Source: CAD feature listing. Evaluate the final solid. Frame: model axes, mm. Face numbers are marked on the shaded views. A direction names the side the tool comes from. Give positions to 0.01 mm unless a question says otherwise; leave off trailing zeros. Order: outer loops, then holes, each group sorted by start corner. A loop starts at its lowest first (then second) coordinate and runs counter-clockwise, first axis right, second up.
from build123d import *

# Parameters (mm, degrees)
SKETCH1_R                           = 66.675
FLANGE_DEPTH                        = 12.7
BOLT_HOLES_D                        = 6.35
BOLT_HOLES_DEPTH                    = 12.7
PIN_HOLES_D                         = 6.35
PIN_HOLES_DEPTH                     = 6.35
PIN_HOLES_TIP                       = 1.907732465
SKETCH2_R                           = 23.8125
SKETCH2_R_2                         = 12.7
FLOW_EXTRUDE_DEPTH                  = 12.7
SKETCH6_R                           = 13.081
SKETCH6_R_2                         = 4.7625
NITROUS_CONNECTION_FLANGE_DEPTH     = 12.7
SKETCH12_R                          = 23.8125
INITIAL_ENTRY_IMPINGING_PLATE_DEPTH = 5.715
SKETCH14_R                          = 23.749
SKETCH15_R                          = 23.8125
SKETCH16_R                          = 12.7
FINAL_FLOW_CUT_DEPTH                = 6.35
TAP_HOLES_FOR_IMPINGING_PLATE_D     = 3.7973
TAP_HOLES_FOR_IMPINGING_PLATE_DEPTH = 12.7
TAP_HOLES_FOR_IMPINGING_PLATE_TIP   = 1.140824014
FLOW_EXTRUDE_FILLET_R               = 3.175
FINAL_FILLET_FOR_HANDLING_R         = 0.635


with BuildPart() as part:
    # Sketch1 → Flange (new body)
    with BuildSketch(Plane(origin=(0, 0, 0), x_dir=(1, 0, 0), z_dir=(0, 1, 0))):
        Circle(SKETCH1_R)
    extrude(amount=FLANGE_DEPTH)

    # Bolt Holes
    with Locations(Plane(origin=(0, 12.7, 0), x_dir=(1, 0, 0), z_dir=(0, 1, 0))):
        with Locations((41.309178157, -41.309178157), (0, -58.42), (-41.309178157, -41.309178157), (-58.42, 0), (-41.309178157, 41.309178157), (0, 58.42), (41.309178157, 41.309178157), (58.42, 0)):
            Hole(BOLT_HOLES_D / 2, depth=BOLT_HOLES_DEPTH)

    # Pin Holes
    with Locations(Plane(origin=(0, 0, 0), x_dir=(-1, 0, 0), z_dir=(0, -1, 0))):
        with Locations((22.356366119, -53.973042289), (-22.356366119, 53.973042289)):
            Hole(PIN_HOLES_D / 2, depth=PIN_HOLES_DEPTH)
            with Locations((0, 0, -(PIN_HOLES_DEPTH + PIN_HOLES_TIP / 2))):  # 118° drill point
                Cone(0, PIN_HOLES_D / 2, PIN_HOLES_TIP, mode=Mode.SUBTRACT)

    # Sketch2 → Flow Extrude (add)
    with BuildSketch(Plane(origin=(0, 12.7, 0), x_dir=(1, 0, 0), z_dir=(0, 1, 0))):
        Circle(SKETCH2_R)
        Circle(SKETCH2_R_2, mode=Mode.SUBTRACT)
    extrude(amount=FLOW_EXTRUDE_DEPTH)

    # Sketch6 → Nitrous Connection Flange (add)
    with BuildSketch(Plane(origin=(0, 25.4, 0), x_dir=(1, 0, 0), z_dir=(0, 1, 0))):
        Circle(SKETCH6_R)
        Circle(SKETCH6_R_2, mode=Mode.SUBTRACT)
    extrude(amount=NITROUS_CONNECTION_FLANGE_DEPTH)

    # Sketch12 → Initial Entry - Impinging Plate (cut)
    with BuildSketch(Plane.XZ):
        Circle(SKETCH12_R)
    extrude(amount=-INITIAL_ENTRY_IMPINGING_PLATE_DEPTH, mode=Mode.SUBTRACT)

    # Sketch14 → Impinging Plate Press Fit Cut section 0
    with BuildSketch(Plane(origin=(0, 6.35, 0), x_dir=(-1, 0, 0), z_dir=(0, -1, 0))):
        Circle(SKETCH14_R)
    # Sketch15 → Impinging Plate Press Fit Cut section 1
    with BuildSketch(Plane.XZ.offset(-5.715)):
        Circle(SKETCH15_R)
    loft(mode=Mode.SUBTRACT)

    # Sketch16 → Final Flow Cut (cut)
    with BuildSketch(Plane.XZ.offset(-6.35)):
        Circle(SKETCH16_R)
    extrude(amount=-FINAL_FLOW_CUT_DEPTH, mode=Mode.SUBTRACT)

    # Tap Holes for Impinging Plate
    with Locations(Plane(origin=(0, 6.35, 0), x_dir=(-1, 0, 0), z_dir=(0, -1, 0))):
        with Locations((0, 17.4625), (17.4625, 0), (0, -17.4625), (-17.4625, 0)):
            Hole(TAP_HOLES_FOR_IMPINGING_PLATE_D / 2, depth=TAP_HOLES_FOR_IMPINGING_PLATE_DEPTH)
            with Locations((0, 0, -(TAP_HOLES_FOR_IMPINGING_PLATE_DEPTH + TAP_HOLES_FOR_IMPINGING_PLATE_TIP / 2))):  # 118° drill point
                Cone(0, TAP_HOLES_FOR_IMPINGING_PLATE_D / 2, TAP_HOLES_FOR_IMPINGING_PLATE_TIP, mode=Mode.SUBTRACT)

    # Flow Extrude Fillet
    flow_extrude_fillet_edges = [part.edges().sort_by_distance(p)[0] for p in [
        (-23.8125, 12.7, 0),
    ]]
    fillet(flow_extrude_fillet_edges, radius=FLOW_EXTRUDE_FILLET_R)

    # Final Fillet for Handling
    final_fillet_for_handling_edges = [part.edges().sort_by_distance(p)[0] for p in [
        (-66.675, 12.7, 0),
        (-23.8125, 25.4, 0),
    ]]
    fillet(final_fillet_for_handling_edges, radius=FINAL_FILLET_FOR_HANDLING_R)


solid = part.part
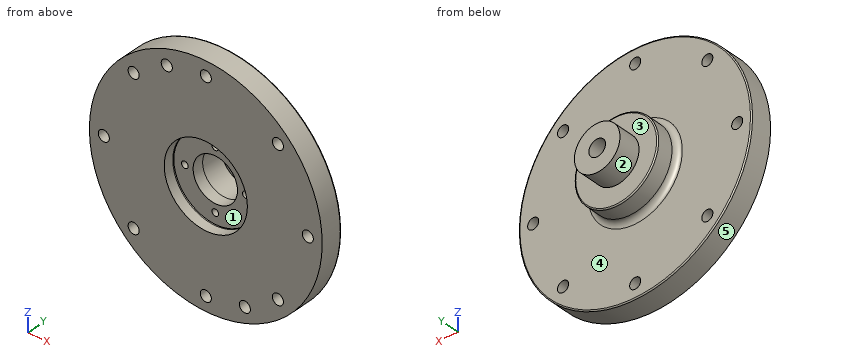
1) Pull-direction query (Z, two-part tool) for the marked faces 1, 2 and 3; classes: +Z half, -Z half, draft (parallel to the pull), parting line (faces both ways), or undercut.
Checks:
face 1: undercut
face 2: parting line
face 3: draft
2) Section query A-A on y = 17.5. Output: boundary loops of the cut face in (x, z) (1 decimal), and give its area (3 significant figures).
Checks:
outline: circle Ø47.6 at (0, 0); hole circle Ø3.8 at (-17.5, 0); hole circle Ø25.4 at (0, 0); hole circle Ø3.8 at (0, -17.5); hole circle Ø3.8 at (0, 17.5); hole circle Ø3.8 at (17.5, 0)
area: 1,230 mm2
3) First-contact query: pin 1 Ø8 at (y, z) = (6, 39) entering from +X; pin 2 Ø8.5 at (x, z) = (-41.31, 41.31) entering from -Y; pin 3 Ø4.5 at (x, z) = (0, -17.46) entering from -Y; pin 4 Ø8 at (x, y) = (-30.5, 9.5) entering from +Z. Flat tips, straight axial feed; report the tip coordinate or a pass-through.
Checks:
pin 1: stops at x = 56.75
pin 2: stops at y = 0
pin 3: stops at y = 6.35
pin 4: stops at z = 61.18
4) Ray query, L1, parallel to Z at x = 0, y = 4.55 (1 decimal); L2, parallel to Y at x = 41, z = -14; L3, parallel to Y at x = 6, z = 5. Return the intervals inside material, ascending.
Checks:
L1: z = -66.7 to -61.6, -55.2 to -23.8, 23.8 to 55.2, 61.6 to 66.7
L2: y = 0 to 12.7
L3: y = 25.4 to 38.1
5) Reachability of the marked faces 4 and 5 from +Z, -Z, +X, -X, +Y, -Y: full face, straight path, thin tool, end or side. Return the list, or none.
Checks:
face 4: +Y
face 5: +Y, -Y
6) Section query B-B on y = 35. Output: boundary loops of the cut face in (x, z) (1 decimal).
Checks:
outline: circle Ø26.2 at (0, 0); hole circle Ø9.5 at (0, 0)
